CAD build for the part. Positions are in the model's coordinates, mm. A direction names the side the tool comes from. Give positions to 0.01 mm unless a question says otherwise; leave off trailing zeros. Loops run counter-clockwise (first coordinate to the right, second up) from the corner with the lowest first, then second, coordinate; pieces in that order, holes last. Notation, with made-up numbers: M 5.5,0.25 L 52.5,0.25 A12 cw 52.5,18.25 Z; hole C 52,-40 d3. An arc over 180 degrees is marked long. One line per question, with ' | ' between items.
```python
from build123d import *

# Parameters (mm, degrees)
SKETCH_1_W                 = 36
SKETCH_1_H                 = 20
EXTRUDE_1_DEPTH            = 15
SKETCH_2_R                 = 2.65
CUT_EXTRUDE_1_DEPTH        = 26.475478406
SKETCH_3_W                 = 12
SKETCH_3_H                 = 8
CUT_EXTRUDE_2_DEPTH        = 31.805843601
SKETCH_5_W                 = 17
SKETCH_5_H                 = 0.5
CUT_EXTRUDE_3_DEPTH        = 31.805843601
SKETCH_6_W                 = 17
SKETCH_6_H                 = 2
CUT_EXTRUDE_4_DEPTH        = 0.6
SKETCH_7_R                 = 4.9
CUT_EXTRUDE_5_DEPTH        = 0.8
SKETCH_8_R                 = 4
CUT_EXTRUDE_6_DEPTH        = 5
HOLE_WIZARD_1_4_28_1_D     = 5.4102
HOLE_WIZARD_1_4_28_1_DEPTH = 5
HOLE_WIZARD_1_4_28_1_TIP   = 1.625388061
SKETCH_11_R                = 0.5
CUT_EXTRUDE_7_DEPTH        = 23.35374689
HOLE_WIZARD_1_4_28_3_D     = 5.4102
HOLE_WIZARD_1_4_28_3_DEPTH = 4
HOLE_WIZARD_1_4_28_3_TIP   = 1.625388061
SKETCH_16_R                = 0.5
CUT_EXTRUDE_8_DEPTH        = 10


with BuildPart() as part:
    # 草图1 → 凸台-拉伸1 (new body)
    with BuildSketch(Plane(origin=(0, 0, 0), x_dir=(1, 0, 0), z_dir=(0, 1, 0))):
        Rectangle(SKETCH_1_W, SKETCH_1_H)
    extrude(amount=EXTRUDE_1_DEPTH)

    # 草图2 → 切除-拉伸1 (cut, through all)
    with BuildSketch(Plane(origin=(0, 15, 0), x_dir=(1, 0, 0), z_dir=(0, 1, 0))):
        with Locations(Location((-12, -2, 0), (0, 0, 270))):
            Circle(SKETCH_2_R)
        with Locations(Location((12, -2, 0), (0, 0, 270))):
            Circle(SKETCH_2_R)
    extrude(amount=-CUT_EXTRUDE_1_DEPTH, mode=Mode.SUBTRACT)

    # 草图3 → 切除-拉伸2 (cut, through all)
    with BuildSketch(Plane.XY.offset(10)):
        with Locations((-12, 11)):
            Rectangle(SKETCH_3_W, SKETCH_3_H)
        with Locations((12, 11)):
            Rectangle(SKETCH_3_W, SKETCH_3_H)
    extrude(amount=-CUT_EXTRUDE_2_DEPTH, mode=Mode.SUBTRACT)

    # 草图5 → 切除-拉伸3 (cut, through all)
    with BuildSketch(Plane.XY.offset(10)):
        with Locations((0, 0.25)):
            Rectangle(SKETCH_5_W, SKETCH_5_H)
    extrude(amount=-CUT_EXTRUDE_3_DEPTH, mode=Mode.SUBTRACT)

    # 草图6 → 切除-拉伸4 (cut)
    with BuildSketch(Plane.XZ.offset(-0.5)):
        with Locations((0, 9)):
            Rectangle(SKETCH_6_W, SKETCH_6_H)
    extrude(amount=-CUT_EXTRUDE_4_DEPTH, mode=Mode.SUBTRACT)

    # 草图7 → 切除-拉伸5 (cut)
    with BuildSketch(Plane.XZ.offset(-0.5)):
        with Locations(Location((0, 2, 0), (0, 0, 270))):
            Circle(SKETCH_7_R)
    extrude(amount=-CUT_EXTRUDE_5_DEPTH, mode=Mode.SUBTRACT)

    # 草图8 → 切除-拉伸6 (cut)
    with BuildSketch(Plane.XZ.offset(-1.3)):
        with Locations(Location((0, 2, 0), (0, 0, 270))):
            Circle(SKETCH_8_R)
    extrude(amount=-CUT_EXTRUDE_6_DEPTH, mode=Mode.SUBTRACT)

    # 1/4-28 螺纹孔1
    with Locations(Plane(origin=(0, 15, 2), x_dir=(0, 0, 1), z_dir=(0, 1, 0))):
        with Locations((0, 0)):
            Hole(HOLE_WIZARD_1_4_28_1_D / 2, depth=HOLE_WIZARD_1_4_28_1_DEPTH)
            with Locations((0, 0, -(HOLE_WIZARD_1_4_28_1_DEPTH + HOLE_WIZARD_1_4_28_1_TIP / 2))):  # 118° drill point
                Cone(0, HOLE_WIZARD_1_4_28_1_D / 2, HOLE_WIZARD_1_4_28_1_TIP, mode=Mode.SUBTRACT)

    # 草图11 → 切除-拉伸7 (cut, through all)
    with BuildSketch(Plane.XZ.offset(-6.3)):
        with Locations(Location((0, 2, 0), (0, 0, 270))):
            Circle(SKETCH_11_R)
    extrude(amount=-CUT_EXTRUDE_7_DEPTH, mode=Mode.SUBTRACT)

    # 1/4-28 螺纹孔3
    with Locations(Plane(origin=(0, 4.7, -10), x_dir=(-1, 0, 0), z_dir=(0, 0, -1))):
        with Locations((0, 0)):
            Hole(HOLE_WIZARD_1_4_28_3_D / 2, depth=HOLE_WIZARD_1_4_28_3_DEPTH)
            with Locations((0, 0, -(HOLE_WIZARD_1_4_28_3_DEPTH + HOLE_WIZARD_1_4_28_3_TIP / 2))):  # 118° drill point
                Cone(0, HOLE_WIZARD_1_4_28_3_D / 2, HOLE_WIZARD_1_4_28_3_TIP, mode=Mode.SUBTRACT)

    # 草图16 → 切除-拉伸8 (cut)
    with BuildSketch(Plane(origin=(0, 0, -10), x_dir=(-1, 0, 0), z_dir=(0, 0, -1))):
        with Locations((0, 4.7)):
            Circle(SKETCH_16_R)
    extrude(amount=-CUT_EXTRUDE_8_DEPTH, mode=Mode.SUBTRACT)


solid = part.part
```
Item 1: Drop flat-ended pins along their axis: P1, Ø12, axis at x = -11.5, z = 0, coming from the -Y side; P2, Ø2.5, axis at y = 11.5, z = 4.5, coming from the +X side; P3, Ø8, axis at x = 12, z = -5.5, coming from the +Y side; P4, Ø3, axis at x = 0, z = 2, coming from the +Y side. Give the stop position or say it passes through.
Conclusion:
P1: y = 0 | P2: x = 6 | P3: y = 7 | P4: y = 9.28
Item 2: Saw through at B-B on x = -12. Give the cut face in (y, z), and give its area (3 significant figures).
Conclusion:
outline: M 0,-10 L 7,-10 L 7,-0.65 L 0,-0.65 Z; M 0,4.65 L 7,4.65 L 7,10 L 0,10 Z | area: 103 mm²
Item 3: Drill centre lines: line 1 along X through (y, z) = (5.2, 2); line 2 along X through (y, z) = (0.7, 2); line 3 along Z through (x, y) = (3, 3). Where is each one in solid material? Low to high. Write a range as [from, to].
Conclusion:
line 1: [-18, -14.65], [-9.35, -4], [4, 9.35], [14.65, 18] | line 2: [-18, -14.65], [-9.35, -4.9], [4.9, 9.35], [14.65, 18] | line 3: [-10, -0.65], [4.65, 10]
Item 4: Saw through at C-C on z = -6.5. Give the cut face in (x, y), and give its area (3 significant figures).
Conclusion:
outline: M -18,0 L -8.5,0 L -8.5,0.5 L 8.5,0.5 L 8.5,0 L 18,0 L 18,7 L 6,7 L 6,15 L -6,15 L -6,7 L -18,7 Z; hole C 0,4.7 d5.41 | area: 317 mm²
Item 5: Saw through at A-A on x = 0. State how many separate pieces and enclosed holes the cut face has, and give its area (3 significant figures).
Conclusion:
separate pieces: 3 | enclosed holes: 0 | area: 179 mm²
Item 6: Saw through at D-D on y = 4.7. Give the cut face in (x, z), and give its area (3 significant figures).
Conclusion:
outline: M -18,-10 L -2.71,-10 L -2.71,-6 L -0.5,-4.68 L -0.5,-1.97 A4 cw long 0.5,-1.97 L 0.5,-4.68 L 2.71,-6 L 2.71,-10 L 18,-10 L 18,10 L -18,10 Z; hole C -12,2 d5.3; hole C 12,2 d5.3 | area: 597 mm²
Item 7: 3-axis set-ups, long thin cutter, end or side, ignore diameter. For faces 4 (the flat face through (-2, 0.5, -3)), 5 (the flat face through (-6, 11, 0)), 6 (the flat face through (8.5, 0.3, 0.1)): which of +Z, -Z, +X, -X, +Y, -Y reach the whole face in a straight line?
Conclusion:
face 4: +Z, -Z, -Y | face 5: +Z, -Z, -X, +Y | face 6: +Z, -Y
Item 8: Mould opens along X. For faces 1 (the flat face through (6, 11, 0)), 2 (the cylindrical face through (1.454, 6.981, -7.972)), 3 (the flat face through (12, 7, -2)) say: pulls with the +X half, pulls with the -X half, needs draft (parallel to the pull), parting line crosses it, or undercut.
Conclusion:
face 1: pulls with the +X half | face 2: undercut | face 3: needs draft
